from build123d import *

# Parameters (mm, degrees)
BOSS_EXTRUDE1_START       = -0.8
BOSS_EXTRUDE1_OUTLINE_R   = 6
BOSS_EXTRUDE1_OUTLINE_R_2 = 2.5
BOSS_EXTRUDE1_DEPTH       = 1
BOSS_EXTRUDE1_START_2     = -9.5
BOSS_EXTRUDE1_2_OUTLINE_R = 2.75
BOSS_EXTRUDE1_2_DEPTH     = 19
BOSS_EXTRUDE1_START_3     = 20.214309477
BOSS_EXTRUDE1_3_OUTLINE_R = 1.25
BOSS_EXTRUDE1_3_DEPTH     = 5
SKETCH2_R                 = 6.25
CUT_EXTRUDE1_DEPTH        = 36.290497761
SKETCH3_R                 = 1.5
CUT_EXTRUDE2_DEPTH        = 10
SKETCH4_R                 = 2.75
SKETCH4_R_2               = 1.5
BOSS_EXTRUDE2_DEPTH       = 19
SKETCH5_W                 = 25.593794746
SKETCH5_H                 = 54.341869273
CUT_EXTRUDE3_DEPTH        = 45.112349032
SKETCH6_W                 = 19
SKETCH6_H                 = 8.728279904
BOSS_EXTRUDE3_DEPTH       = 1.568762114
SKETCH7_W                 = 4.505283746
SKETCH7_H                 = 5.968681608
CUT_EXTRUDE4_DEPTH        = 40.377309908


with BuildPart() as part:
    # Boss-Extrude1: read off the stored shape, not the designer's step
    # Boss-Extrude1 outline → Boss-Extrude1 (new body)
    with BuildSketch(Plane(origin=(0, 0, 24.414309477), x_dir=(-1, 0, 0), z_dir=(0, 0, -1)).offset(BOSS_EXTRUDE1_START)):
        with Locations((0, 13.101553709)):
            Circle(BOSS_EXTRUDE1_OUTLINE_R)
        with Locations((0, 13.101553709)):
            Circle(BOSS_EXTRUDE1_OUTLINE_R_2, mode=Mode.SUBTRACT)
    extrude(amount=BOSS_EXTRUDE1_DEPTH)

    # Boss-Extrude1 2 outline → Boss-Extrude1 2 (add)
    with BuildSketch(Plane.YZ.offset(BOSS_EXTRUDE1_START_2)):
        with BuildLine():
            Line((30.808082296, 25.214309477), (-4.594884555, 25.214309477))
            ThreePointArc((-4.594884555, 25.214309477), (-6.157718154, 25.077579254), (-7.673065845, 24.671543064))
            Line((-7.673065845, 24.671543064), (-24.384342131, 18.58913592))
            ThreePointArc((-24.384342131, 18.58913592), (-26.882991431, 12.373899853), (-20.43432651, 10.560855883))
            Line((-20.43432651, 10.560855883), (-7.673065845, 18.658005573))
            ThreePointArc((-7.673065845, 18.658005573), (-5.104992299, 19.817354852), (-2.315454789, 20.214309477))
            Line((-2.315454789, 20.214309477), (30.808082296, 20.214309477))
            Line((30.808082296, 20.214309477), (30.808082296, 25.214309477))
        make_face()
        with Locations((-22.845251486, 14.360519126)):
            Circle(BOSS_EXTRUDE1_2_OUTLINE_R, mode=Mode.SUBTRACT)
    extrude(amount=BOSS_EXTRUDE1_2_DEPTH)

    # Boss-Extrude1 3 outline → Boss-Extrude1 3 (cut)
    with BuildSketch(Plane.XY.offset(BOSS_EXTRUDE1_START_3)):
        with BuildLine():
            ThreePointArc((-9.5, 25.808082296), (-8.035533906, 29.343616202), (-4.5, 30.808082296))
            Line((-4.5, 30.808082296), (-9.5, 30.808082296))
            Line((-9.5, 30.808082296), (-9.5, 25.808082296))
        make_face()
        with BuildLine():
            Line((9.5, 30.808082296), (4.5, 30.808082296))
            ThreePointArc((4.5, 30.808082296), (8.035533906, 29.343616202), (9.5, 25.808082296))
            Line((9.5, 25.808082296), (9.5, 30.808082296))
        make_face()
        with Locations((5, 26.808082296)):
            Circle(BOSS_EXTRUDE1_3_OUTLINE_R)
        with Locations((-5, 26.808082296)):
            Circle(BOSS_EXTRUDE1_3_OUTLINE_R)
    extrude(amount=BOSS_EXTRUDE1_3_DEPTH, mode=Mode.SUBTRACT)

    # Boss-Extrude1 4 outline → Boss-Extrude1 4 (revolve, cut)
    with BuildSketch(Plane.XZ.offset(-13.101553709)):
        Polygon((6, 20.714309477), (6, 24.214309477), (2.5, 24.214309477), (2.5, 25.214309477), (0, 25.214309477), (0, 20.214309477), (6.5, 20.214309477), align=None)
    revolve(axis=Axis((0, 13.101553709, 0), (0, 0, 1)), mode=Mode.SUBTRACT)

    # Sketch2 → Cut-Extrude1 (cut, through all)
    with BuildSketch(Plane(origin=(0, 0, 24.214309477), x_dir=(-1, 0, 0), z_dir=(0, 0, -1))):
        with Locations((0, 13.101553709)):
            Circle(SKETCH2_R)
    extrude(amount=CUT_EXTRUDE1_DEPTH, mode=Mode.SUBTRACT)

    # Sketch3 → Cut-Extrude2 (cut)
    with BuildSketch(Plane.XY.offset(25.214309477)):
        with Locations((-5, 26.808082296)):
            Circle(SKETCH3_R)
        with Locations((5, 26.808082296)):
            Circle(SKETCH3_R)
    extrude(amount=-CUT_EXTRUDE2_DEPTH, mode=Mode.SUBTRACT)

    # Sketch4 → Boss-Extrude2 (add)
    with BuildSketch(Plane.ZY.offset(9.5)):
        with Locations((14.360519126, -22.845251486)):
            Circle(SKETCH4_R)
        with Locations((14.360519126, -22.845251486)):
            Circle(SKETCH4_R_2, mode=Mode.SUBTRACT)
    extrude(amount=-BOSS_EXTRUDE2_DEPTH)

    # Sketch5 → Cut-Extrude3 (cut, through all)
    with BuildSketch(Plane(origin=(9.5, 0, 0), x_dir=(0, 0, -1), z_dir=(1, 0, 0))):
        with Locations((-21.9386431, 9.463333989)):
            Rectangle(SKETCH5_W, SKETCH5_H)
    extrude(amount=-CUT_EXTRUDE3_DEPTH, mode=Mode.SUBTRACT)

    # Sketch6 → Boss-Extrude3 (add)
    with BuildSketch(Plane(origin=(0, -17.707600648, 0), x_dir=(1, 0, 0), z_dir=(0, 1, 0))):
        with Locations((0, -16.655131129)):
            Rectangle(SKETCH6_W, SKETCH6_H)
    extrude(amount=BOSS_EXTRUDE3_DEPTH)

    # Sketch7 → Cut-Extrude4 (cut, through all)
    with BuildSketch(Plane(origin=(9.5, 0, 0), x_dir=(0, 0, -1), z_dir=(1, 0, 0))):
        with Locations((-22.271912954, -19.123179338)):
            Rectangle(SKETCH7_W, SKETCH7_H)
    extrude(amount=-CUT_EXTRUDE4_DEPTH, mode=Mode.SUBTRACT)


solid = part.part
CAD build for the part. Positions are in the model's coordinates, mm. Round coordinates to 2 decimals unless told otherwise and drop trailing zeros. Write each loop counter-clockwise with the first axis right and the second up, starting at its lowest first coordinate (ties: lowest second). Pieces come first, ordered by that corner, then holes.
(1) Drop flat-ended pins along their axis: P1, Ø1.5, axis at x = 7, y = -25.5, coming from the -Z side; P2, Ø6, axis at x = 6.5, y = -24, coming from the +Z side; P3, Ø1.7, axis at x = -0.5, y = -16.5, coming from the -Z side. Give the stop position or say it passes through.
(2) Slice it at C-C, the plane z = 16.5. Write the cut outline in (x, y).
(3) Slice it at B-B, the plane y = -18.5. Write the cut outline in (x, z).
(4) Probe line 1 along Z through (x, y) = (2.75, -23.75); line 2 along Z through (x, y) = (-4, -22.25); line 3 along Y through (x, z) = (7.5, 13). List the from-to ranges inside material, lowest first.
(5) Slice it at A-A, the plane x = -1. Write the cut outline in (y, z), and give its area (3 significant figures).
(6) Mould opens along Z. For faces 1 (the face through (-0.13, -23.76, 13.17)), 2 (the face through (0, -17, 12.291)), 3 (the face through (0, -16.139, 16)) say: pulls with the +Z half, pulls with the -Z half, needs draft (parallel to the pull), parting line crosses it, or undercut.
From the geometry:
1. P1: stops at z = 10.28
1. P2: stops at z = 19.82
1. P3: stops at z = 12.29
2. outline: (-9.5, -26.8) - (9.5, -26.8) - (9.5, -16.14) - (-9.5, -16.14) - close
3. outline: (-9.5, 11.79) - (9.5, 11.79) - (9.5, 20.02) - (-9.5, 20.02) - close
4. line 1: z = 9.95 to 13.16, 15.56 to 18.82
4. line 2: z = 9.9 to 12.98, 15.74 to 19.37
4. line 3: y = -27.13 to -23.48, -22.21 to -16.14
5. outline: (-24.38, 18.59) arc R4.5 ccw (long way) to (-20.43, 10.56) - (-17.71, 12.29) - (-16.14, 12.29) - (-16.14, 20.02) - (-20.46, 20.02) - close; hole circle Ø3 at (-22.85, 14.36)
5. area: 83.4 mm2
6. face 1: undercut
6. face 2: pulls with the -Z half
6. face 3: needs draft
